Autodesk Fusion 360 part; units mm, degrees
sketch "Sketch1" plane through (0, 0, 0) normal (0, 1, 0) x (1, 0, 0)
  line L0 (2.5, -2.5) -> (27.5, -2.5)
  arc A0 (27.5, -2.5) -> (27.5, 2.5) centre (27.5, 0) ccw
  arc A1 (2.5, 2.5) -> (2.5, -2.5) centre (2.5, 0) ccw
  line L1 (0, 0) -> (30, 0) construction
  line L2 (15, 2.5) -> (15, 10) construction
  line L3 (15, 2.5) -> (15, -7) construction
  arc A2 (18, 2.5) -> (12, 2.5) centre (15, 2.5) ccw
  line L4 (27.5, 2.5) -> (18, 2.5)
  line L5 (12, 2.5) -> (2.5, 2.5)
  point P0 (15, 0)
  dimension "d2" = 6
  dimension "d3" = 30
  dimension "d5" = 5
sketch "Sketch2" plane through (0, 0, 0) normal (0, 1, 0) x (1, 0, 0)
  line L0 (30, 10) -> (30, -30)
  line L1 (92.5, 20) -> (-62.5, 20)
  line L2 (-62.5, 20) -> (-62.5, -20)
  line L3 (-62.5, -20) -> (92.5, -20)
  line L4 (92.5, -20) -> (92.5, 20)
  line L5 (92.5, 20) -> (-62.5, -20) construction
  line L6 (-62.5, 20) -> (92.5, -20) construction
  point P0 (15, 0)
  point P1 (15, 0)
  dimension "d7" = 40
  dimension "d10" = 40
  dimension "d11" = 155
extrude "Extrude1" add sketch "Sketch2" sketch "Sketch1" along normal blind 0.6 of sketch 2
extrude "Extrude2" cut sketch "Sketch1" along normal up to surface (0.6 mm away)
sketch "Sketch3" plane through (0, 0.6, 0) normal (0, 1, 0) x (-1, 0, 0)
  line L0 (-27.5, 2.5) -> (-2.5, 2.5)
  arc A0 (-2.5, -2.5) -> (-2.5, 2.5) centre (-2.5, 0) ccw
  line L1 (-2.5, -2.5) -> (-12, -2.5)
  arc A1 (-18, -2.5) -> (-12, -2.5) centre (-15, -2.5) ccw
  line L2 (-18, -2.5) -> (-27.5, -2.5)
  arc A2 (-27.5, 2.5) -> (-27.5, -2.5) centre (-27.5, 0) ccw
  line L3 (-92.5, 20) -> (-92.5, -20)
  line L4 (-92.5, -20) -> (62.5, -20)
  line L5 (62.5, -20) -> (62.5, 20)
  line L6 (62.5, 20) -> (-92.5, 20)
  line L7 (-2.5, 2.5) -> (-27.5, 2.5)
  arc A3 (-27.5, 2.5) -> (-27.5, -2.5) centre (-27.5, 0) ccw
  line L8 (-27.5, -2.5) -> (-18, -2.5)
  arc A4 (-18, -2.5) -> (-12, -2.5) centre (-15, -2.5) ccw
  line L9 (-12, -2.5) -> (-2.5, -2.5)
  arc A5 (-2.5, -2.5) -> (-2.5, 2.5) centre (-2.5, 0) ccw
  line L10 (-92.5, -20) -> (-92.5, 20)
  line L11 (-92.5, 20) -> (62.5, 20)
  line L12 (62.5, 20) -> (62.5, -20)
  line L13 (62.5, -20) -> (-92.5, -20)
  line L14 (-15, -5.5) -> (-102, -5.5) construction
  line L15 (-15, -5.5) -> (63, -5.5) construction
  dimension "d17" = 8
equation "d7 = Linear Dimension-3"
equation "breite = 155 mm"
equation "d10 = Linear Dimension-3"
equation "d11 = breite"
equation "dicke = 0.6 mm"
equation "d13 = dicke"
Could you check a few things on this model? Use its own coordinates, in mm. A direction names the side the tool comes from. Coordinates: 2 decimals unless noted, no trailing zeros. Write each loop counter-clockwise with the first axis right and the second up, starting at its lowest first coordinate (ties: lowest second). Pieces come first, ordered by that corner, then holes. Notation, with made-up numbers: (57.5, 22.25) - (76.5, 22.25) arc R30 cw to (76.5, 60.25) - close; hole circle Ø6 at (89.25, 47). An arc over 180 degrees is marked (long way). Write item = value, one per line.
1) For faces 1 (the cylindrical face through (30, 0.3, -0.1)), 2 (the flat face through (14, 0, 4)), which set-ups out of +Z, -Z, +X, -X, +Y, -Y let a thin tool reach every point of the face, with its end or its side?
Result set:
face_1 = +Y, -Y
face_2 = +Z, -Z, +X, -X, -Y
2) Suppose I cut it at B-B on y = 0.5. Please give me the cut outline in (x, z), plus the area to 3 significant figures.
Result set:
outline = (-62.5, -20) - (92.5, -20) - (92.5, 20) - (-62.5, 20) - close; hole (2.5, -2.5) - (12, -2.5) arc R3 ccw to (18, -2.5) - (27.5, -2.5) arc R2.5 ccw to (27.5, 2.5) - (2.5, 2.5) arc R2.5 ccw to start
area = 6,040 mm2
3) Suppose I cut it at A-A on x = 10.5. Please give me the cut outline in (y, z).
Result set:
outline = (0, -20) - (0.6, -20) - (0.6, -2.5) - (0, -2.5) - close; (0, 2.5) - (0.6, 2.5) - (0.6, 20) - (0, 20) - close
4) Please list where these lines run through material, in increasing order: line 1 (Z direction, x = 23, y = 0.5); line 2 (Z direction, x = 14, y = 0.3); line 3 (X direction, y = 0.4, z = -3). Write a range as [from, to].
Result set:
line_1 = [-20, -2.5], [2.5, 20]
line_2 = [-20, -5.33], [2.5, 20]
line_3 = [-62.5, 12.04], [17.96, 92.5]
